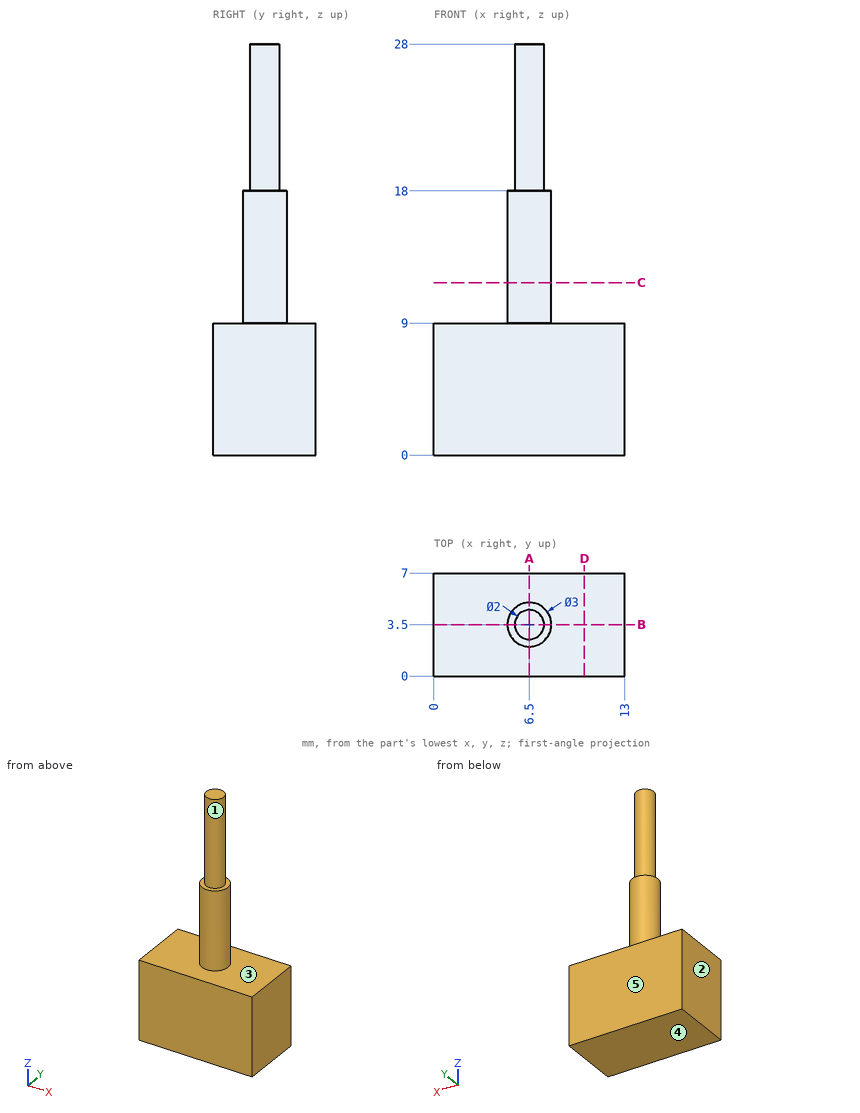
For this review, use the dimensioned drawing (mm, ordinates from the lowest corner) and the shaded views. A direction names the side the tool comes from. Round coordinates to 2 decimals unless told otherwise and drop trailing zeros. Order: outer loops, then holes, each group sorted by start corner. A loop starts at its lowest first (then second) coordinate and runs counter-clockwise, first axis right, second up. Notation, with made-up numbers: (38.5, 22.25) -> (89.5, 22.25) arc R18 cw to (89.5, 52.25) -> close; hole circle Ø3 at (74, 46.5). An arc over 180 degrees is marked (long way). One line per item, written item: value. Start each with the question number.
Q1. Take a section at B-B (y = 3.5). Write out the cut boundary in (x, z), and give its area (3 significant figures).
Q2. Machinability: for the marked faces 1 and 2, which of the approach directions +Z, -Z, +X, -X, +Y, -Y give a long, thin tool a straight path to every point of the face, cutting with its end or side? Answer none if there is none.
Q3. Take a section at C-C (z = 11.75). Write out the cut boundary in (x, y).
Q4. Wall thickness on line 1 (Z direction, x = 4.5, y = 1.5); line 2 (Z direction, x = 6.25, y = 2.5); line 3 (X direction, y = 4, z = 16): over which ranges is each line inside the solid? List them lowest first.
Q5. Mouldability with a two-part tool opening along Z and no side actions: class the marked faces 3, 4 and 5 as released by +Z, released by -Z, zero draft, split by the parting line, or undercut.
Q6. Take a section at A-A (x = 6.5). Write out the cut boundary in (y, z).
Q7. Take a section at D-D (x = 10.25). Write out the cut boundary in (y, z).
Q8. Clearance check with flat-ended pins moving along their axes: pin 1 Ø1.5 at (y, z) = (5.5, 16.5) entering from -X; pin 2 Ø1 at (x, z) = (7.5, 20.5) entering from +Y; pin 3 Ø1.5 at (y, z) = (5, 22) entering from -X. State where each tip first meets the part, or that it passes through.
Reported:
1. outline: (0, 0) -> (13, 0) -> (13, 9) -> (8, 9) -> (8, 18) -> (7.5, 18) -> (7.5, 28) -> (5.5, 28) -> (5.5, 18) -> (5, 18) -> (5, 9) -> (0, 9) -> close
1. area: 164 mm2
2. face 1: +Z
2. face 2: +Z, -Z, -X, +Y, -Y
3. outline: circle Ø3 at (6.5, 3.5)
4. line 1: z = 0 to 9
4. line 2: z = 0 to 18
4. line 3: x = 5.09 to 7.91
5. face 3: released by +Z
5. face 4: released by -Z
5. face 5: zero draft
6. outline: (0, 0) -> (7, 0) -> (7, 9) -> (5, 9) -> (5, 18) -> (4.5, 18) -> (4.5, 28) -> (2.5, 28) -> (2.5, 18) -> (2, 18) -> (2, 9) -> (0, 9) -> close
7. outline: (0, 0) -> (7, 0) -> (7, 9) -> (0, 9) -> close
8. pin 1: stops at x = 5.67
8. pin 2: stops at y = 4.37
8. pin 3: stops at x = 5.84
